from build123d import *

# Parameters (mm, degrees)
F0_W     = 20
F0_H     = 20
F1_DEPTH = 20
F2_W     = 3
F2_H     = 4
F2_W_2   = 15
F2_H_2   = 3
F3_DEPTH = 20.001
F4_W     = 8
F4_H     = 3
F5_DEPTH = 20.001
F6_W     = 1.5
F6_H     = 4
F7_DEPTH = 3


with BuildPart() as f1:
    # F0 (on Top) → F1 (new body)
    with BuildSketch(Plane.XY):
        Rectangle(F0_W, F0_H)
    extrude(amount=F1_DEPTH)

    # F2 (on face) → F3 (cut, through all)
    with BuildSketch(Plane.XZ.offset(10)):
        with Locations((-5.98057, 4)):
            Rectangle(F2_W, F2_H)
        with Locations((0.01943, 4)):
            Rectangle(F2_W, F2_H)
        with Locations((6.01943, 4)):
            Rectangle(F2_W, F2_H)
        with Locations((0.01943, 15.283564)):
            Rectangle(F2_W_2, F2_H_2)
    extrude(amount=-F3_DEPTH, mode=Mode.SUBTRACT)

    # F4 (on face) → F5 (cut, through all)
    with BuildSketch(Plane.YZ.offset(10)):
        with Locations((-3.447752, 9.344094)):
            Rectangle(F4_W, F4_H)
    extrude(amount=-F5_DEPTH, mode=Mode.SUBTRACT)

    # F6 (on face) → F7 (cut, through all)
    with BuildSketch(Plane.YZ.offset(-1.48057)):
        with Locations((-7.75, 4)):
            Rectangle(F6_W, F6_H)
        with Locations((-1.14, 4)):
            Rectangle(F6_W, F6_H)
        with Locations((5.47, 4)):
            Rectangle(F6_W, F6_H)
    extrude(amount=-F7_DEPTH, mode=Mode.SUBTRACT)


solid = f1.part
The model under review builds one solid part; all positions refer to its coordinate system, in mm. A direction names the side the tool comes from. Round coordinates to 2 decimals unless told otherwise and drop trailing zeros. Order: outer loops, then holes, each group sorted by start corner. A loop starts at its lowest first (then second) coordinate and runs counter-clockwise, first axis right, second up. Notation, with made-up numbers: (31.5, -27) -> (68.5, -27) arc R8 ccw to (68.5, -15) -> close; hole circle Ø9 at (88.25, 64). An arc over 180 degrees is marked (long way). Write item = value, one per line. Start each with the question number.
Item 1: Consider section A-A on x = 5.5. Write out the cut boundary in (y, z), plus the area to 3 significant figures.
Item 2: Mouldability with a two-part tool opening along Z and no side actions: class faces 4 (the face through (0, 0, 13.784)), 5 (the face through (0, -10, 10)), 6 (the face through (0, 0, 20)) as released by +Z, released by -Z, zero draft, split by the parting line, or undercut.
Item 3: For faces 1 (the face through (-10, 2, 10)), 2 (the face through (-3, -0.39, 4)), 3 (the face through (-1.481, 2, 4)), list the 3-axis set-ups (+Z, -Z, +X, -X, +Y, -Y) from which the entire face can be reached by the end or side of a thin tool; tool diameter is ignored.
Item 4: Consider section C-C on x = -2.25. Write out the cut boundary in (y, z), plus the area to 3 significant figures.
Item 5: For line 1 along X through (y, z) = (7, 4); line 2 along Y through (x, z) = (-2, 2.25); line 3 along Z through (x, y) = (-7, 7), list the stretches that pass through material, from the lowest coordinate up.
Item 6: Consider section D-D on y = -0.75. Write out the cut boundary in (x, z).
Item 7: Consider section B-B on y = -4. Write out the cut boundary in (x, z).
Conclusion:
q1.outline = (-10, 0) -> (10, 0) -> (10, 2) -> (-10, 2) -> close; (-10, 6) -> (10, 6) -> (10, 13.78) -> (-10, 13.78) -> close; (-10, 16.78) -> (10, 16.78) -> (10, 20) -> (-10, 20) -> close; hole (-7.45, 7.84) -> (0.55, 7.84) -> (0.55, 10.84) -> (-7.45, 10.84) -> close
q1.area = 236 mm2
q2.face_4 = undercut
q2.face_5 = zero draft
q2.face_6 = released by +Z
q3.face_1 = +Z, -Z, -X, +Y, -Y
q3.face_2 = none
q3.face_3 = +Y, -Y
q4.outline = (-10, 0) -> (10, 0) -> (10, 13.78) -> (-10, 13.78) -> close; (-10, 16.78) -> (10, 16.78) -> (10, 20) -> (-10, 20) -> close; hole (-8.5, 2) -> (-7, 2) -> (-7, 6) -> (-8.5, 6) -> close; hole (-7.45, 7.84) -> (0.55, 7.84) -> (0.55, 10.84) -> (-7.45, 10.84) -> close; hole (-1.89, 2) -> (-0.39, 2) -> (-0.39, 6) -> (-1.89, 6) -> close; hole (4.72, 2) -> (6.22, 2) -> (6.22, 6) -> (4.72, 6) -> close
q4.area = 298 mm2
q5.line_1 = -10 to -7.48, -4.48 to -1.48, 1.52 to 4.52, 7.52 to 10
q5.line_2 = -10 to -8.5, -7 to -1.89, -0.39 to 4.72, 6.22 to 10
q5.line_3 = 0 to 2, 6 to 13.78, 16.78 to 20
q6.outline = (-10, 0) -> (10, 0) -> (10, 7.84) -> (-10, 7.84) -> close; (-10, 10.84) -> (10, 10.84) -> (10, 20) -> (-10, 20) -> close; hole (-7.48, 2) -> (1.52, 2) -> (1.52, 6) -> (-7.48, 6) -> close; hole (-7.48, 13.78) -> (7.52, 13.78) -> (7.52, 16.78) -> (-7.48, 16.78) -> close; hole (4.52, 2) -> (7.52, 2) -> (7.52, 6) -> (4.52, 6) -> close
q7.outline = (-10, 0) -> (10, 0) -> (10, 7.84) -> (-10, 7.84) -> close; (-10, 10.84) -> (10, 10.84) -> (10, 20) -> (-10, 20) -> close; hole (-7.48, 2) -> (-4.48, 2) -> (-4.48, 6) -> (-7.48, 6) -> close; hole (-7.48, 13.78) -> (7.52, 13.78) -> (7.52, 16.78) -> (-7.48, 16.78) -> close; hole (-1.48, 2) -> (1.52, 2) -> (1.52, 6) -> (-1.48, 6) -> close; hole (4.52, 2) -> (7.52, 2) -> (7.52, 6) -> (4.52, 6) -> close
